Autodesk Inventor part; units mm, degrees
sketch "スケッチ1" plane through (0, 0, 0) normal (0, 0, 1) x (1, 0, 0)
  circle A0 centre (0, 0) radius 5.25
  circle A1 centre (0, 0) radius 7.05
  dimension "d0" = 10.5
  dimension "d1" = 14.1
extrude "押し出し1" add sketch "スケッチ1" along normal blind 10 and the other way blind 3.5 contours A0 | A1
sketch "スケッチ2" plane through (0, 0, 0) normal (0, 0, 1) x (1, 0, 0)
  line L0 (-25, 5) -> (0, 5)
  line L1 (0, 5) -> (0, -5)
  line L2 (0, -5) -> (-25, -5)
  line L3 (-25, -5) -> (-25, 5)
  point P0 (0, 0)
  dimension "d4" = 25
  dimension "d5" = 5
  dimension "d6" = 10
extrude "押し出し2" add sketch "スケッチ2" along normal mid plane 3
sketch "スケッチ5" plane through (0, 0, -3.5) normal (0, 0, -1) x (-1, 0, 0)
  circle A0 centre (0, 0) radius 5.35
  dimension "d21" = 10.7
extrude "押し出し5" cut sketch "スケッチ5" against normal through all
sketch "スケッチ9" plane through (0, 0, 0) normal (0, 0, 1) x (1, 0, 0)
  line L0 (8.4285, -5) -> (-7.6033, -5)
  line L1 (-7.6033, 5) -> (8.4285, 5)
  arc A0 (4.9702, -5) -> (4.9702, 5) centre (0, 0) ccw
  arc A1 (-4.9702, 5) -> (-4.9702, -5) centre (0, 0) ccw
  arc A2 (8.4285, -5) -> (8.4285, 5) centre (0, 0) ccw
  arc A3 (-7.6033, 5) -> (-7.6033, -5) centre (0, 0) ccw
  dimension "d74" = 5
  dimension "d75" = 5
  dimension "d79" = 9.8
extrude "押し出し9" add sketch "スケッチ9" along normal mid plane 3 contours L0 A0 L1 A2
sketch "スケッチ6" plane through (0, 0, -3.5) normal (0, 0, -1) x (-1, 0, 0)
  line L0 (7.2132, -2.9681) -> (-7.7309, 1.0362)
  line L1 (-7.2132, 2.9681) -> (7.7309, -1.0362)
  line L2 (11.6181, 0) -> (-15.1574, 0)
  arc A0 (7.2132, -2.9681) -> (7.7309, -1.0362) centre (0, 0) ccw
  arc A1 (-7.2132, 2.9681) -> (-7.7309, 1.0362) centre (0, 0) ccw
  point P0 (-11.3323, 4.0718)
  dimension "d24" = 1
  dimension "d43" = 15
  dimension "d64" = 1
  dimension "d65" = 7.8
  dimension "d66" = 7.8
extrude "押し出し6" cut sketch "スケッチ6" against normal blind 3.5
move faces "移動4" translate (0, 0, 2) faces at (5.6485, 3.107, -3.5) (-3.1586, -5.6105, -3.5)
ref_plane "作業平面1" through (0, 0, 0) normal (-0.258819, 0.9659258, 0) x (0, 0, 1)
chamfer "面取り1" distance 0.5 angle 45 4 edges at (-7.7309, -1.0362, -0.75) (7.7309, 1.0362, -0.75) (7.2132, 2.9681, -0.75) (-7.2132, -2.9681, -0.75)
chamfer "面取り2" distance 1.2 angle 45 2 edges at (5.1677, 1.3847, 0) (-5.1677, -1.3847, 0)
move faces "移動5" translate (0, 0, -1.25) faces at (-6.7087, -1.8554, 0) (6.7087, 1.8554, 0)
properties part number "HbThumbProximalPhalanxBase01" material "ABS プラスチック"
Geometry check sheet. Reference: the model listing, model coordinates, mm. A direction names the side the tool comes from. Give positions to 0.01 mm unless a question says otherwise; leave off trailing zeros. Loops run counter-clockwise (first coordinate to the right, second up) from the corner with the lowest first, then second, coordinate; pieces in that order, holes last. Notation, with made-up numbers: (12.5, -27) - (56.5, -27) arc R4 cw to (56.5, -20) - close; hole circle Ø6 at (32, -11.5). An arc over 180 degrees is marked (long way). Use CSV: the item, a comma, the result in double quotes. Start each with the question number.
Q1. Section check A-A, the plane x = 0. Record the cut outline in (y, z), and give its area (3 significant figures).
Q2. Section check D-D, the plane x = -4. Record the cut outline in (y, z).
Q3. Section check B-B, the plane y = 0. Record the cut outline in (x, z), and give its area (3 significant figures).
Q4. Scan lines: probe 1 along Y at (x, z) = (0, 3.25); probe 2 along Z at (x, y) = (-11.5, 1.25). Record each from-to range of solid material in increasing order. Write a range as from..to.
Q5. Section check C-C, the plane z = 5. Record the cut outline in (x, y).
Q6. Go/stop test with flat-tipped pins: pin 1 Ø3 at (x, z) = (3.5, 1) entering from +Y; pin 2 Ø3 at (x, y) = (1.5, -1.5) entering from -Z; pin 3 Ø5 at (y, z) = (-3.5, 2.5) entering from +X; pin 4 Ø6 at (x, z) = (-9, 2) entering from -Y. Record where each tip stops, or that it passes through.
Q7. Access from +Z, -Z, +X, -X, +Y, -Y to the whole of each face (thin tool, end or side, straight path). Record for faces 5 (the face through (-15, 5, 0)), 6 (the face through (6.1, 1.65, 0.23)), 7 (the face through (6.512, -2.7, 4.33)), 8 (the face through (7, -5, 0)).
Q8. Release check for a two-part mould opening along Y. For faces 1 (the face through (7, 5, 0)), 2 (the face through (-5.575, -2.529, -0.469)), 3 (the face through (-12, 0, -1.5)), 4 (the face through (6.1, 0.6, -0.5)) record: +Y half, -Y half, draft (parallel to the pull), parting line (faces both ways), or undercut.
Findings below:
1,outline,"(-7.05, -1.5) - (-5.35, -1.5) - (-5.35, 10) - (-7.05, 10) - close; (5.35, -1.5) - (7.05, -1.5) - (7.05, 10) - (5.35, 10) - close"
1,area,"39.1 mm^2"
2,outline,"(-5.81, -1.5) - (-3.55, -1.5) - (-3.55, 10) - (-5.81, 10) - close; (3.55, -1.5) - (5.81, -1.5) - (5.81, 10) - (3.55, 10) - close"
3,outline,"(-25, -1.5) - (-5.35, -1.5) - (-5.35, 10) - (-7.05, 10) - (-7.05, 1.5) - (-25, 1.5) - close; (5.35, -1.5) - (9.8, -1.5) - (9.8, 1.5) - (7.05, 1.5) - (7.05, 10) - (5.35, 10) - close"
3,area,"101 mm^2"
4,probe 1,"y = -7.05..-5.35, 5.35..7.05"
4,probe 2,"z = -1.5..1.5"
5,outline,"circle Ø14.1 at (0, 0); hole circle Ø10.7 at (0, 0)"
6,pin 1,"stops at y = 6.76"
6,pin 2,"passes through"
6,pin 3,"stops at x = 9.73"
6,pin 4,"stops at y = -5"
7,face 5,"+Z, -Z, -X, +Y"
7,face 6,"-Z"
7,face 7,"+Z"
7,face 8,"+Z, -Z, +X, -Y"
8,face 1,"+Y half"
8,face 2,"undercut"
8,face 3,"draft"
8,face 4,"undercut"
